Read the model definition and answer for the solid it produces. Units are mm, in the model's axes. Face numbers are marked on the shaded views. A direction names the side the tool comes from. Give positions to 0.01 mm unless a question says otherwise; leave off trailing zeros. Write each loop counter-clockwise with the first axis right and the second up, starting at its lowest first coordinate (ties: lowest second). Pieces come first, ordered by that corner, then holes. Notation, with made-up numbers: (1.25, 39.25) -> (36.25, 39.25) arc R29 cw to (36.25, 71.25) -> close; hole circle Ø6 at (78, 29.25). An arc over 180 degrees is marked (long way). Use a Markdown table: item, result.
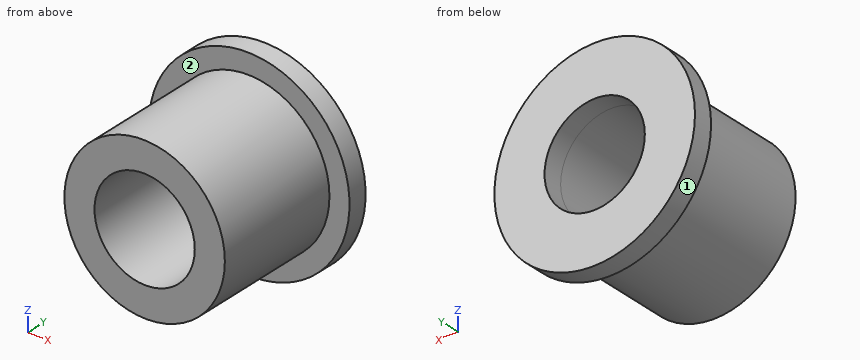
from build123d import *

# Parameters (mm, degrees)
F0_R     = 8
F0_R_2   = 5
F1_DEPTH = 13
F2_R     = 10
F2_R_2   = 5
F3_DEPTH = 2


with BuildPart() as f1:
    # F0 (on Front) → F1 (new body)
    with BuildSketch(Plane.XZ):
        Circle(F0_R)
        Circle(F0_R_2, mode=Mode.SUBTRACT)
    extrude(amount=F1_DEPTH)

    # F2 (on face) → F3 (join)
    with BuildSketch(Plane(origin=(0, 0, 0), x_dir=(-1, 0, 0), z_dir=(0, 1, 0))):
        Circle(F2_R)
        Circle(F2_R_2, mode=Mode.SUBTRACT)
    extrude(amount=F3_DEPTH)


solid = f1.part
Item 1: A cutting plane is placed at C-C (y = -5.5). Give the vertices of the cut face in (x, z), then the cut area to 3 significant figures.
Return value:
| item | result |
|---|---|
| outline | circle Ø16 at (0, 0); hole circle Ø10 at (0, 0) |
| area | 123 mm^2 |
Item 2: Straight lines are drawn through the part: line 1 along Z through (x, y) = (0, 0.45); line 2 along Z through (x, y) = (0, -6.25); line 3 along X through (y, z) = (-1.25, 4.5). For each, find the intervals that lie inside material, in ascending order. Write a range as [from, to].
Return value:
| item | result |
|---|---|
| line 1 | [-10, -5], [5, 10] |
| line 2 | [-8, -5], [5, 8] |
| line 3 | [-6.61, -2.18], [2.18, 6.61] |
Item 3: A cutting plane is placed at D-D (z = 7.25). Give the vertices of the cut face in (x, y), then the cut area to 3 significant figures.
Return value:
| item | result |
|---|---|
| outline | (-6.89, 0) -> (-3.38, 0) -> (-3.38, -13) -> (3.38, -13) -> (3.38, 0) -> (6.89, 0) -> (6.89, 2) -> (-6.89, 2) -> close |
| area | 115 mm^2 |
Item 4: A cutting plane is placed at A-A (z = 0). Give the vertices of the cut face in (x, y).
Return value:
| item | result |
|---|---|
| outline | (-10, 0) -> (-8, 0) -> (-8, -13) -> (-5, -13) -> (-5, 2) -> (-10, 2) -> close; (5, -13) -> (8, -13) -> (8, 0) -> (10, 0) -> (10, 2) -> (5, 2) -> close |
Item 5: A tool of negligible diameter and unlimited length cuts with its end or side. For the marked faces 1 and 2, from which of +Z, -Z, +X, -X, +Y, -Y can it reach the whole face along a straight path? Write none if from no direction.
Return value:
| item | result |
|---|---|
| face 1 | +Y, -Y |
| face 2 | -Y |
Item 6: A cutting plane is placed at B-B (x = 0). Give the vertices of the cut face in (y, z).
Return value:
| item | result |
|---|---|
| outline | (-13, -8) -> (0, -8) -> (0, -10) -> (2, -10) -> (2, -5) -> (-13, -5) -> close; (-13, 5) -> (2, 5) -> (2, 10) -> (0, 10) -> (0, 8) -> (-13, 8) -> close |
Item 7: Each of these flat-tipped pins is pushed along its axis until it touches: P1, Ø1.5, axis at y = -0.5, z = -4, coming from the -X side; P2, Ø2, axis at y = -2, z = -2, coming from the +X side; P3, Ø4, axis at y = -3.5, z = 7.5, coming from the +X side. Where does it stop, or does it pass through?
Return value:
| item | result |
|---|---|
| P1 | x = -9.39 |
| P2 | x = 7.94 |
| P3 | x = 5.81 |
